Verification items for the finished model (mm, model axes). Face numbers are marked on the shaded views. Round coordinates to 2 decimals unless told otherwise and drop trailing zeros. Loops run counter-clockwise (first coordinate to the right, second up) from the corner with the lowest first, then second, coordinate; pieces in that order, holes last. Notation, with made-up numbers: M 7.5,22 L 47.5,22 A13 cw 47.5,33 Z; hole C -7.5,42 d7. An arc over 180 degrees is marked long. Answer as CSV lines item,"result".
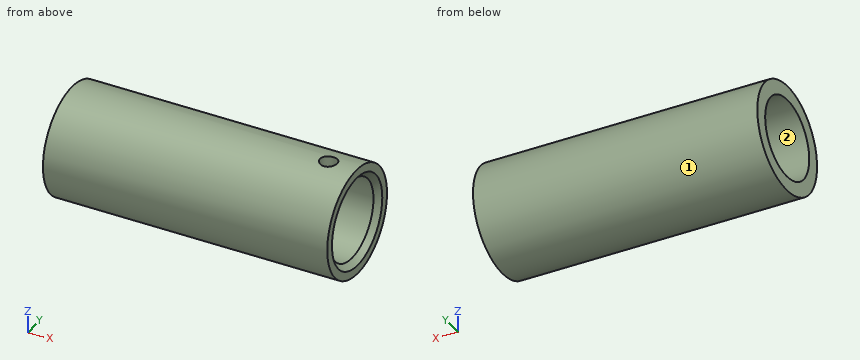
```python
from build123d import *

# Parameters (mm, degrees)
F0_R     = 19
F0_R_2   = 14
F1_DEPTH = 100
F4_SIZE2 = 2
F4_SIZE  = 2
F5_D     = 6
F5_DEPTH = 15


with BuildPart() as f1:
    # F0 (on Right) → F1 (new body)
    with BuildSketch(Plane.YZ):
        Circle(F0_R)
        Circle(F0_R_2, mode=Mode.SUBTRACT)
    extrude(amount=F1_DEPTH)

    # F4
    f4_edges = [f1.edges().sort_by_distance(p)[0] for p in [
        (100, -14, 0),
    ]]
    chamfer(f4_edges, length=F4_SIZE, length2=F4_SIZE2)

    # F5
    with Locations(Plane.XY.offset(19)):
        with Locations((90, 0)):
            Hole(F5_D / 2, depth=F5_DEPTH)


solid = f1.part
```
1) Material ranges on probe 1 along Z at (x, y) = (76, 0); probe 2 along Z at (x, y) = (59, -1.5); probe 3 along Z at (x, y) = (91, 0), recorded low to high.
Here are the results:
probe 1,"z = -19 to -14, 14 to 19"
probe 2,"z = -18.94 to -13.92, 13.92 to 18.94"
probe 3,"z = -19 to -14"
2) Section check B-B (y = 0). Record the cut outline in (x, z), plus the area to 3 significant figures.
Here are the results:
outline,"M 0,-19 L 100,-19 L 100,-16 L 98,-14 L 0,-14 Z; M 0,14 L 87,14 L 87,19 L 0,19 Z; M 93,14 L 98,14 L 100,16 L 100,19 L 93,19 Z"
area,"966 mm^2"
3) Draft check along Y on the marked faces 1 and 2. Enter one of: +Y half, -Y half, draft (parallel to the pull), parting line (faces both ways), or undercut.
Here are the results:
face 1,"parting line"
face 2,"undercut"
4) Section check A-A (z = 0). Record the cut outline in (x, y).
Here are the results:
outline,"M 0,-19 L 100,-19 L 100,-16 L 98,-14 L 0,-14 Z; M 0,14 L 98,14 L 100,16 L 100,19 L 0,19 Z"
5) Go/stop test with flat-tipped pins: pin 1 (8 mm diameter, centred on x = 82, y = 11, fed in from +Z); pin 2 (4 mm diameter, centred on x = 59, z = 12.5, fed in from +Y); pin 3 (4 mm diameter, centred on x = 78.5, y = 2.5, fed in from -Z). Record where each tip stops, or that it passes through.
Here are the results:
pin 1,"stops at z = 17.66"
pin 2,"stops at y = 15.84"
pin 3,"stops at z = -18.99"
6) Section check C-C (x = 84.5). Record the cut outline in (y, z).
Here are the results:
outline,"C 0,0 d38; hole C 0,0 d28"
